Read the model definition and answer for the solid it produces. Units are mm, in the model's axes. Face numbers are marked on the shaded views. A direction names the side the tool comes from. Coordinates: 2 decimals unless noted, no trailing zeros. Order: outer loops, then holes, each group sorted by start corner. A loop starts at its lowest first (then second) coordinate and runs counter-clockwise, first axis right, second up. Notation, with made-up numbers: M -36,-20 L 6,-20 A18 ccw 6,6 Z; hole C -23,72.5 d1. An arc over 180 degrees is marked long. Put each result on its own line as item: value.
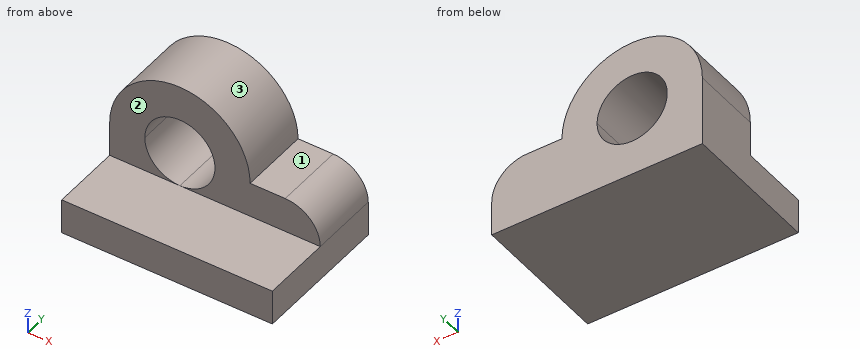
from build123d import *

# Parameters (mm, degrees)
F1_DEPTH = 40
F2_DEPTH = 20


with BuildPart() as f1:
    # F0 (on Front) → F1 (new body)
    with BuildSketch(Plane.XZ):
        with BuildLine():
            ThreePointArc((37.3205080757, 10), (30, 2.6794919243), (20, 0))
            Line((20, 0), (60, 0))
            Line((60, 0), (60, 10))
            Line((60, 10), (37.3205080757, 10))
        make_face()
        with BuildLine():
            Line((0, 10), (0, 0))
            Line((0, 0), (20, 0))
            ThreePointArc((20, 0), (10, 2.6794919243), (2.6794919243, 10))
            Line((2.6794919243, 10), (0, 10))
        make_face()
        with BuildLine():
            ThreePointArc((2.6794919243, 10), (10, 2.6794919243), (20, 0))
            ThreePointArc((20, 0), (30, 2.6794919243), (37.3205080757, 10))
            Line((37.3205080757, 10), (19.9999999466, 10))
            Line((19.9999999466, 10), (2.6794919243, 10))
        make_face()
    extrude(amount=F1_DEPTH)

    # F0 (on Front) → F2 (join)
    with BuildSketch(Plane.XZ):
        with BuildLine():
            Line((0, 10), (0, 0))
            Line((0, 0), (20, 0))
            ThreePointArc((20, 0), (10, 2.6794919243), (2.6794919243, 10))
            Line((2.6794919243, 10), (0, 10))
        make_face()
        with BuildLine():
            Line((0, 20), (0, 10))
            Line((0, 10), (2.6794919243, 10))
            ThreePointArc((2.6794919243, 10), (0.6814834742, 14.8236190979), (0, 20))
        make_face()
        with BuildLine():
            ThreePointArc((37.3205080757, 10), (30, 2.6794919243), (20, 0))
            Line((20, 0), (60, 0))
            Line((60, 0), (60, 10))
            Line((60, 10), (37.3205080757, 10))
        make_face()
        with BuildLine():
            ThreePointArc((2.6794919243, 10), (10, 2.6794919243), (20, 0))
            ThreePointArc((20, 0), (30, 2.6794919243), (37.3205080757, 10))
            Line((37.3205080757, 10), (19.9999999466, 10))
            Line((19.9999999466, 10), (2.6794919243, 10))
        make_face()
        with BuildLine():
            ThreePointArc((0, 20), (0.6814834742, 14.8236190979), (2.6794919243, 10))
            Line((2.6794919243, 10), (19.9999999466, 10))
            ThreePointArc((19.9999999466, 10), (12.9289321693, 12.928932207), (10, 20))
            Line((10, 20), (0, 20))
        make_face()
        with BuildLine():
            ThreePointArc((40, 20), (20, 40), (0, 20))
            Line((0, 20), (10, 20))
            ThreePointArc((10, 20), (20, 30), (30, 20))
            Line((30, 20), (40, 20))
        make_face()
        with BuildLine():
            ThreePointArc((40, 20), (39.3185165258, 14.8236190979), (37.3205080757, 10))
            Line((37.3205080757, 10), (60, 10))
            ThreePointArc((60, 10), (57.0710678119, 17.0710678119), (50, 20))
            Line((50, 20), (40, 20))
        make_face()
        with BuildLine():
            Line((19.9999999466, 10), (37.3205080757, 10))
            ThreePointArc((37.3205080757, 10), (39.3185165258, 14.8236190979), (40, 20))
            Line((40, 20), (30, 20))
            ThreePointArc((30, 20), (27.071067793, 12.9289321693), (19.9999999466, 10))
        make_face()
    extrude(amount=F2_DEPTH)


solid = f1.part
Q1. Find section B-B on x = 22. Write down the section's boundary in (y, z), plus the area to 3 significant figures.
Answers below:
outline: M -40,0 L 0,0 L 0,10.2 L -20,10.2 L -20,10 L -40,10 Z; M -20,29.8 L 0,29.8 L 0,39.9 L -20,39.9 Z
area: 606 mm^2
Q2. A tool of negligible diameter and unlimited length cuts with its end or side. For the marked faces 1, 2 and 3, from which of +Z, -Z, +X, -X, +Y, -Y can it reach the whole face along a straight path? Write none if from no direction.
Answers below:
face 1: +Z, +X, +Y, -Y
face 2: +Z, +X, -X, -Y
face 3: +Z, +Y, -Y
Q3. Given pin 1 (4 mm diameter, centred on y = -9.5, z = 30, fed in from +X); pin 2 (4 mm diameter, centred on x = 21.5, y = -10.5, fed in from +Z); pin 3 (3 mm diameter, centred on x = 46, y = -14.5, fed in from +Z), each flat-ended and moving along its own axis, determine where each tip first touches the part or whether it passes through.
Answers below:
pin 1: stops at x = 38.33
pin 2: stops at z = 40
pin 3: stops at z = 20
Q4. Find section A-A on y = -18.5. Write down the section's boundary in (x, z).
Answers below:
outline: M 0,0 L 60,0 L 60,10 A10 ccw 50,20 L 40,20 A20 ccw 0,20 Z; hole C 20,20 d20
Q5. Find section D-D on y = -24. Write down the section's boundary in (x, z), plus the area to 3 significant figures.
Answers below:
outline: M 0,0 L 60,0 L 60,10 L 0,10 Z
area: 600 mm^2
Q6. Consider line 1 along Y through (x, z) = (35, 13.5); line 2 along Z through (x, y) = (20, -21.5); line 3 along X through (y, z) = (-16, 23.5). Determine where each line is inside the solid, lowest interval first.
Answers below:
line 1: y = -20 to 0
line 2: z = 0 to 10
line 3: x = 0.31 to 10.63, 29.37 to 39.69
Q7. Find section C-C on z = 27. Write down the section's boundary in (x, y) (3 decimals).
Answers below:
outline: M 1.265,-20 L 12.859,-20 L 12.859,0 L 1.265,0 Z; M 27.141,-20 L 38.735,-20 L 38.735,0 L 27.141,0 Z
